The model under review builds one solid part; all positions refer to its coordinate system, in mm. Face numbers are marked on the shaded views. Coordinates: 2 decimals unless noted, no trailing zeros. Write each loop counter-clockwise with the first axis right and the second up, starting at its lowest first coordinate (ties: lowest second). Pieces come first, ordered by that corner, then holes.
1) For P1, Ø2, axis at x = 9, y = -6, coming from the -Z side; P2, Ø2, axis at y = -11, z = -9, coming from the +X side; P3, Ø1, axis at x = 2.5, z = 9, coming from the +Y side, all flat-tipped, find the tip position at first contact; note any pin that passes through.
2) For line 1 (Z direction, x = 12.25, y = 0); line 2 (X direction, y = 0.5, z = 3), list the stretches that pass through material, from the lowest coordinate up.
3) Add section A-A, the plane z = 0. State the section outline as (x, y) points, then the cut area to 3 significant figures.
4) Mouldability with a two-part tool opening along Z and no side actions: class the marked faces 1, 2 and 3 as released by +Z, released by -Z, zero draft, split by the parting line, or undercut.
5) Add section D-D, the plane x = 8. State the section outline as (y, z) points, then the cut area to 3 significant figures.
6) Add section C-C, the plane x = 16. State the section outline as (y, z) points, then the cut area to 3 significant figures.
from build123d import *

# Parameters (mm, degrees)
SCHIZZO1_R                   = 9.5
SCHIZZO1_R_2                 = 8
ESTRUSIONE_ESTRUSIONE1_DEPTH = 20
SCHIZZO2_R                   = 15
ESTRUSIONE_ESTRUSIONE2_DEPTH = 5
RACCORDO1_R                  = 5


with BuildPart() as part:
    # Schizzo1 → Estrusione-Estrusione1 (new body)
    with BuildSketch(Plane(origin=(0, 0, 0), x_dir=(0, 0, -1), z_dir=(1, 0, 0))):
        Circle(SCHIZZO1_R)
        Circle(SCHIZZO1_R_2, mode=Mode.SUBTRACT)
    extrude(amount=ESTRUSIONE_ESTRUSIONE1_DEPTH)

    # Schizzo2 → Estrusione-Estrusione2 (add)
    with BuildSketch(Plane(origin=(0, 0, 0), x_dir=(0, 0, -1), z_dir=(1, 0, 0))):
        Circle(SCHIZZO2_R)
    extrude(amount=ESTRUSIONE_ESTRUSIONE2_DEPTH)

    # Raccordo1
    raccordo1_edges = [part.edges().sort_by_distance(p)[0] for p in [
        (5, 0, 9.5),
    ]]
    fillet(raccordo1_edges, radius=RACCORDO1_R)


solid = part.part
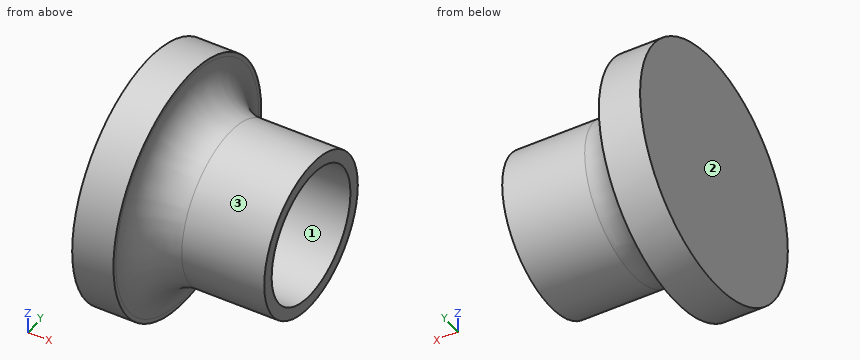
Geometry results:
1. P1: stops at z = -8.27
1. P2: stops at x = 5.17
1. P3: stops at y = 12.36
2. line 1: z = -9.5 to -8, 8 to 9.5
2. line 2: x = 0 to 5
3. outline: (0, -15) - (5, -15) - (5, -14.5) arc R5 cw to (10, -9.5) - (20, -9.5) - (20, -8) - (5, -8) - (5, 8) - (20, 8) - (20, 9.5) - (10, 9.5) arc R5 cw to (5, 14.5) - (5, 15) - (0, 15) - close
3. area: 206 mm2
4. face 1: undercut
4. face 2: zero draft
4. face 3: split by the parting line
5. outline: circle Ø19.83 at (0, 0); hole circle Ø16 at (0, 0)
5. area: 108 mm2
6. outline: circle Ø19 at (0, 0); hole circle Ø16 at (0, 0)
6. area: 82.5 mm2
